Check sheet for the modelled part. Datum: model origin and axes. Units: mm. Round coordinates to 2 decimals unless told otherwise and drop trailing zeros. Write each loop counter-clockwise with the first axis right and the second up, starting at its lowest first coordinate (ties: lowest second). Pieces come first, ordered by that corner, then holes. Notation, with made-up numbers: (55.5, 28.5) - (96.5, 28.5) arc R18 ccw to (96.5, 47.5) - close; hole circle Ø2 at (33.5, -37.5). An arc over 180 degrees is marked (long way). Answer as a JSON object with one key per item and string values. Group by question number.
Item 1: Gauge pin test, flat ends, axial feed: P1, Ø1, axis at x = -11, y = -16, coming from the +Z side; P2, Ø2, axis at x = 19.5, y = -1.5, coming from the -Z side; P3, Ø2, axis at x = 11, y = 10.5, coming from the +Z side; P4, Ø5, axis at x = -16, y = -4, coming from the -Z side. Record the tip position at first contact, or that the pin passes through.
Item 2: Thickness scan on line 1 (Y direction, x = -32.5, z = 0); line 2 (Y direction, x = 19.5, z = 6.5); line 3 (Z direction, x = 3.5, y = -11). Record the ranges inside material, lowest first.
Item 3: Sectioned sample at C-C on y = -18.5. Record the boundary of the cut face in (x, z).
Item 4: Sectioned sample at D-D on x = -37.5. Record the boundary of the cut face in (y, z).
Item 5: Sectioned sample at B-B on x = 25. Record the boundary of the cut face in (y, z).
Item 6: Release check for a two-part mould opening along X. For faces 1 (the cylindrical face through (40.31, -1.86, -14.18)), 2 (the cylindrical face through (-40.5, -17.8, -0.1)), 3 (the flat face through (44.5, 0, 0)), 4 (the flat face through (-38, -21, 0)) record: pulls with the +X half, pulls with the -X half, needs draft (parallel to the pull), parting line crosses it, or undercut.
Item 7: Sectioned sample at A-A on z = 0. Record the boundary of the cut face in (x, y), plus the area to 3 significant figures.
```python
from build123d import *

# Parameters (mm, degrees)
SKETCH1_W           = 84
SKETCH1_H           = 15
SKETCH3_R           = 3
BOSS_EXTRUDE1_DEPTH = 21
SKETCH4_W           = 5
SKETCH4_H           = 15
SKETCH5_W           = 1.6
SKETCH5_H           = 0.7


with BuildPart() as part:
    # Sketch1 → Revolve1 (revolve)
    with BuildSketch(Plane.XY):
        with Locations((-2.5, 7.5)):
            Rectangle(SKETCH1_W, SKETCH1_H)
    revolve(axis=Axis((39.5, 0, 0), (-1, 0, 0)))

    # Sketch2 → Cut-Revolve1 (revolve, cut)
    with BuildSketch(Plane.XY):
        Polygon((-44.5, 13.5), (-43, 15), (-44.5, 15), align=None)
    revolve(axis=Axis((77, 0, 0), (-1, 0, 0)), mode=Mode.SUBTRACT)

    # Sketch3 → Boss-Extrude1 (add)
    with BuildSketch(Plane(origin=(0, 0, 0), x_dir=(1, 0, 0), z_dir=(0, 1, 0))):
        with Locations((-37.5, 0)):
            Circle(SKETCH3_R)
    extrude(amount=-BOSS_EXTRUDE1_DEPTH)

    # Sketch4 → Revolve2 (revolve)
    with BuildSketch(Plane.XY):
        with Locations((42, 7.5)):
            Rectangle(SKETCH4_W, SKETCH4_H)
    revolve(axis=Axis((44.5, 0, 0), (-1, 0, 0)))

    # Sketch5 → Cut-Revolve2 (revolve, cut)
    with BuildSketch(Plane.XY):
        with Locations((40.3, 14.65)):
            Rectangle(SKETCH5_W, SKETCH5_H)
    revolve(axis=Axis((77, 0, 0), (-1, 0, 0)), mode=Mode.SUBTRACT)

    # Sketch6 → Cut-Revolve3 (revolve, cut)
    with BuildSketch(Plane.XY):
        Polygon((43, 15), (44.5, 13.5), (44.5, 15), align=None)
    revolve(axis=Axis((77, 0, 0), (-1, 0, 0)), mode=Mode.SUBTRACT)


solid = part.part
```
Completed:
{
 "1": {"P1": "through", "P2": "z = -14.99", "P3": "z = 11.61", "P4": "z = -14.92"},
 "2": {"line 1": "-15 to 15", "line 2": "-13.52 to 13.52", "line 3": "-10.2 to 10.2"},
 "3": {"outline": "circle Ø6 at (-37.5, 0)"},
 "4": {"outline": "(-21, -3) - (-14.7, -3) arc R15 ccw (long way) to (-14.7, 3) - (-21, 3) - close"},
 "5": {"outline": "circle Ø30 at (0, 0)"},
 "6": {"face 1": "undercut", "face 2": "parting line crosses it", "face 3": "pulls with the +X half", "face 4": "needs draft"},
 "7": {"outline": "(-44.5, -13.5) - (-43, -15) - (-40.5, -15) - (-40.5, -21) - (-34.5, -21) - (-34.5, -15) - (39.5, -15) - (39.5, -14.3) - (41.1, -14.3) - (41.1, -15) - (43, -15) - (44.5, -13.5) - (44.5, 13.5) - (43, 15) - (41.1, 15) - (41.1, 14.3) - (39.5, 14.3) - (39.5, 15) - (-43, 15) - (-44.5, 13.5) - close", "area": "2,700 mm²"}
}
